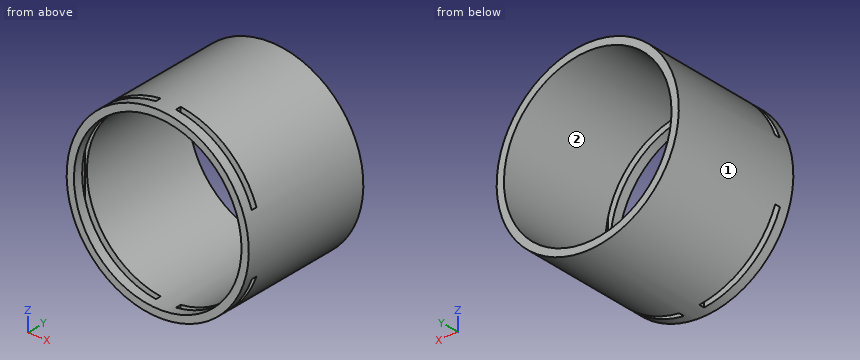
from build123d import *

# Parameters (mm, degrees)
SKETCH1_R               = 60.071
BOSS_EXTRUDE1_DEPTH     = 88.9
SKETCH2_R               = 55.245
CUT_EXTRUDE1_DEPTH      = 123.964466745
CUT_EXTRUDE4_DEPTH      = 123.964466745
CUT_EXTRUDE4_DEPTH_BACK = 123.964466745
SKETCH6_W               = 50.038
SKETCH6_H               = 3.683


with BuildPart() as part:
    # Sketch1 → Boss-Extrude1 (new body)
    with BuildSketch(Plane(origin=(0, 0, 0), x_dir=(1, 0, 0), z_dir=(0, 1, 0))):
        with Locations(Location((0, 0, 0), (0, 0, 270))):
            Circle(SKETCH1_R)
    extrude(amount=BOSS_EXTRUDE1_DEPTH)

    # Sketch2 → Cut-Extrude1 (cut, through all)
    with BuildSketch(Plane(origin=(0, 88.9, 0), x_dir=(1, 0, 0), z_dir=(0, 1, 0))):
        with Locations(Location((0, 0, 0), (0, 0, 270))):
            Circle(SKETCH2_R)
    extrude(amount=-CUT_EXTRUDE1_DEPTH, mode=Mode.SUBTRACT)

    # Sketch6 → Cut-Extrude4 (cut, two sides: drawn at the far end of the back side and taken through both)
    with BuildSketch(Plane.XY.offset(-CUT_EXTRUDE4_DEPTH_BACK)):
        with Locations((-31.623, 8.1915)):
            Rectangle(SKETCH6_W, SKETCH6_H)
        with Locations((31.623, 8.1915)):
            Rectangle(SKETCH6_W, SKETCH6_H)
    extrude(amount=CUT_EXTRUDE4_DEPTH + CUT_EXTRUDE4_DEPTH_BACK, mode=Mode.SUBTRACT)


solid = part.part
Geometry check sheet. Reference: the model listing, model coordinates, mm. Face numbers are marked on the shaded views. Coordinates: 2 decimals unless noted, no trailing zeros. Loops run counter-clockwise (first coordinate to the right, second up) from the corner with the lowest first, then second, coordinate; pieces in that order, holes last. Notation, with made-up numbers: (50.5, -13) - (92.5, -13) arc R23 cw to (92.5, 26) - close; hole circle Ø11 at (38.5, -37). An arc over 180 degrees is marked (long way). Use one line per item in the form item = value. Start each with the question number.
Item 1: Section check A-A, the plane z = 0. Enter the section's corners in (x, y) (3 decimals).
Item 2: Gauge pin test, flat ends, axial feed: pin 1 (1.8 mm diameter, centred on y = 9, z = -57.5, fed in from +X); pin 2 (1 mm diameter, centred on x = -20.5, y = 32.5, fed in from +Z); pin 3 (4 mm diameter, centred on y = 20, z = 8.5, fed in from +X). Record the tip position at first contact, or that the pin passes through.
Item 3: Section check D-D, the plane x = 23.5. Enter the section's corners in (y, z).
Item 4: Thickness scan on probe 1 along Y at (x, z) = (54, 15.5); probe 2 along Z at (x, y) = (-1, 20); probe 3 along X at (y, z) = (54, 0) (3 decimals). Record the ranges inside material, lowest first.
Item 5: Mould release check, pull along X, two halves, no side actions. Record for the marked faces 1 and 2: +X half, -X half, draft (parallel to the pull), parting line (faces both ways), or undercut.
Item 6: Section check B-B, the plane x = 0. Enter the section's corners in (y, z) (3 decimals), and give its area (3 significant figures).
Item 7: Section check C-C, the plane y = 8. Enter the section's corners in (x, z) (3 decimals).
Computed:
q1.outline = (-60.071, 0) - (-55.245, 0) - (-55.245, 6.35) - (-56.642, 6.35) - (-56.642, 10.033) - (-55.245, 10.033) - (-55.245, 88.9) - (-60.071, 88.9) - close; (55.245, 0) - (60.071, 0) - (60.071, 88.9) - (55.245, 88.9) - (55.245, 10.033) - (56.642, 10.033) - (56.642, 6.35) - (55.245, 6.35) - close
q2.pin_1 = 6.6
q2.pin_2 = 56.64
q2.pin_3 = 59.72
q3.outline = (0, -55.28) - (6.35, -55.28) - (6.35, -50) - (0, -50) - close; (0, 50) - (6.35, 50) - (6.35, 55.28) - (0, 55.28) - close; (10.03, -55.28) - (88.9, -55.28) - (88.9, -50) - (10.03, -50) - close; (10.03, 50) - (88.9, 50) - (88.9, 55.28) - (10.03, 55.28) - close
q4.probe_1 = 0 to 6.35, 10.03 to 88.9
q4.probe_2 = -60.06 to -55.24, 55.24 to 60.06
q4.probe_3 = -60.071 to -55.245, 55.245 to 60.071
q5.face_1 = parting line
q5.face_2 = undercut
q6.outline = (0, -60.071) - (88.9, -60.071) - (88.9, -55.245) - (0, -55.245) - close; (0, 55.245) - (88.9, 55.245) - (88.9, 60.071) - (0, 60.071) - close
q6.area = 858 mm2
q7.outline = (-56.642, -20.005) - (-56.642, 20.005) arc R60.071 ccw to start; (-6.604, -59.707) arc R60.071 ccw to (6.604, -59.707) - (6.604, -54.849) arc R55.245 cw to (-6.604, -54.849) - close; (-6.604, 54.849) arc R55.245 cw to (6.604, 54.849) - (6.604, 59.707) arc R60.071 ccw to (-6.604, 59.707) - close; (56.642, -20.005) arc R60.071 ccw to (56.642, 20.005) - close
